from build123d import *

# Parameters (mm, degrees)
F0_R     = 2.7
F0_R_2   = 4.5
F0_R_3   = 2.6
F0_R_4   = 1.6
F1_DEPTH = 3.2
F2_R     = 10


with BuildPart() as f1:
    # F0 (on Front) → F1 (new body)
    with BuildSketch(Plane.XZ):
        with BuildLine():
            Line((75, -12.5), (75, 12.5))
            Line((75, 12.5), (-5, 12.5))
            Line((-5, 12.5), (-5, 37.5))
            Line((-5, 37.5), (-40, 37.5))
            Line((-40, 37.5), (-40, 12.5))
            Line((-40, 12.5), (-60, 12.5))
            ThreePointArc((-60, 12.5), (-72.5, 0), (-60, -12.5))
            Line((-60, -12.5), (75, -12.5))
        make_face()
        with Locations((-10, -2.5)):
            Circle(F0_R, mode=Mode.SUBTRACT)
        with Locations((-60, 0)):
            Circle(F0_R_2, mode=Mode.SUBTRACT)
        with Locations((60, 0)):
            Circle(F0_R_3, mode=Mode.SUBTRACT)
        with Locations((-22.5, 25)):
            Circle(F0_R_4, mode=Mode.SUBTRACT)
    extrude(amount=F1_DEPTH)

    # F2
    f2_edges = [f1.edges().sort_by_distance(p)[0] for p in [
        (75, -1.6, 12.5),
        (75, -1.6, -12.5),
    ]]
    fillet(f2_edges, radius=F2_R)


solid = f1.part
Design review of the part built by this model. Coordinates are the model's own, in mm. A direction names the side the tool comes from. Coordinates: 2 decimals unless noted, no trailing zeros. Order: outer loops, then holes, each group sorted by start corner. A loop starts at its lowest first (then second) coordinate and runs counter-clockwise, first axis right, second up. Notation, with made-up numbers: (15.25, 31) -> (33.25, 31) arc R27 ccw to (33.25, 69) -> close; hole circle Ø4 at (9, 47.25). An arc over 180 degrees is marked (long way). Use one line per item in the form item = value. Start each with the question number.
(1) Add section A-A on z = 25. State the section outline as (x, y) points, plus the area to 3 significant figures.
(2) Insertion check: pin 1 (1.9 mm diameter, centred on x = -22.5, z = 25, fed in from +Y); pin 2 (1.6 mm diameter, centred on y = -2, z = 24.5, fed in from -X); pin 3 (1.6 mm diameter, centred on x = 35.5, y = -1, fed in from +Z); pin 4 (1 mm diameter, centred on y = -1, z = 23.5, fed in from +X). Each pin has a flat end and moves straight along its axis. Give the tip position at first contact, or say it passes through.
(3) Add section D-D on z = 31.5. State the section outline as (x, y) points, plus the area to 3 significant figures.
(4) For probe 1 along Z at (x, y) = (60, -2.15); probe 2 along X at (y, z) = (-3.05, -1.5); probe 3 along Z at (x, y) = (-22.5, -2.1), list the stretches that pass through material, from the lowest coordinate up.
(5) The part is to be moulded in two halves that separate along Z. For faces 1 (the cylindrical face through (-7.425, -1.578, -1.689)), 2 (the flat face through (75, -2, 0)), 3 (the cylindrical face through (-55.708, -1.578, 1.352)), 4 (the flat face through (2, -2, -12.5)), say which applies: +Z half, -Z half, draft (parallel to the pull), parting line (faces both ways), or undercut.
(6) Add section C-C on y = -2.6. State the section outline as (x, z) points, plus the area to 3 significant figures.
(7) Add section B-B on x = 60. State the section outline as (y, z) points, plus the area to 3 significant figures.
(8) For faces 5 (the flat face through (-50, -2, 12.5)), 6 (the flat face through (-5, -2, 25)), 7 (the cylindrical face through (57.4, -1.6, 0.1)), list the 3-axis set-ups (+Z, -Z, +X, -X, +Y, -Y) from which the entire face can be reached by the end or side of a thin tool; tool diameter is ignored.
Answer block:
q1.outline = (-40, -3.2) -> (-24.1, -3.2) -> (-24.1, 0) -> (-40, 0) -> close; (-20.9, -3.2) -> (-5, -3.2) -> (-5, 0) -> (-20.9, 0) -> close
q1.area = 102 mm²
q2.pin_1 = through
q2.pin_2 = -40
q2.pin_3 = 12.5
q2.pin_4 = -5
q3.outline = (-40, -3.2) -> (-5, -3.2) -> (-5, 0) -> (-40, 0) -> close
q3.area = 112 mm²
q4.probe_1 = -12.5 to -2.6, 2.6 to 12.5
q4.probe_2 = -72.41 to -64.24, -55.76 to -12.51, -7.49 to 57.88, 62.12 to 75
q4.probe_3 = -12.5 to 23.4, 26.6 to 37.5
q5.face_1 = undercut
q5.face_2 = draft
q5.face_3 = undercut
q5.face_4 = -Z half
q6.outline = (-60, -12.5) -> (65, -12.5) arc R10 ccw to (75, -2.5) -> (75, 2.5) arc R10 ccw to (65, 12.5) -> (-5, 12.5) -> (-5, 37.5) -> (-40, 37.5) -> (-40, 12.5) -> (-60, 12.5) arc R12.5 ccw to start; hole circle Ø9 at (-60, 0); hole circle Ø3.2 at (-22.5, 25); hole circle Ø5.4 at (-10, -2.5); hole circle Ø5.2 at (60, 0)
q6.area = 4,340 mm²
q7.outline = (-3.2, -12.5) -> (0, -12.5) -> (0, -2.6) -> (-3.2, -2.6) -> close; (-3.2, 2.6) -> (0, 2.6) -> (0, 12.5) -> (-3.2, 12.5) -> close
q7.area = 63.4 mm²
q8.face_5 = +Z, -X, +Y, -Y
q8.face_6 = +Z, +X, +Y, -Y
q8.face_7 = +Y, -Y
